Here's how the part is built. I have some questions about the finished solid (model axes, mm). Round coordinates to 2 decimals unless told otherwise and drop trailing zeros. Write each loop counter-clockwise with the first axis right and the second up, starting at its lowest first coordinate (ties: lowest second). Pieces come first, ordered by that corner, then holes. Notation, with made-up numbers: (23.25, -6) - (81.25, -6) arc R30 cw to (81.25, 27) - close; hole circle Ø8 at (84, 18.25). An arc over 180 degrees is marked (long way). One line per item, written item: value. Start each with the question number.
Item 1: Imagine slicing it at A-A, the plane y = 534. Please give me the cut outline in (x, z), then the cut area to 3 significant figures.
Item 2: For P1, Ø0.6, axis at x = 197.5, z = 0.5, coming from the +Y side; P2, Ø0.6, axis at y = 543.5, z = 1.5, coming from the -X side, each with a flat end and sliding along its axis, tell me the tip position at first contact or that it passes through.
Item 3: If I drill on line 1 (X direction, y = 539.5, z = 1.1); line 2 (X direction, y = 452.5, z = 0.6); line 3 (Y direction, x = 190.5, z = 1.75), over which ranges is the centre line in solid material (lowest first)?
```python
from build123d import *

# Parameters (mm, degrees)
EXTRUDE_1_DEPTH = 2


with BuildPart() as part:
    # 草图1 → 凸台-拉伸1 (new body)
    with BuildSketch(Plane.XY):
        with BuildLine():
            Line((244.967841267, 542.393386476), (173.531139847, 542.393386476))
            Line((173.531139847, 542.393386476), (173.531139847, 544.404513771))
            Line((173.531139847, 544.404513771), (166.427186265, 544.404513771))
            Line((166.427186265, 544.404513771), (166.427186265, 523.784577737))
            Line((166.427186265, 523.784577737), (165.125301121, 523.784577737))
            Line((165.125301121, 523.784577737), (165.381520735, 509.161664861))
            add(Edge.make_bspline(
                [(165.381520735, 509.161664861), (166.398492196, 499.581380375), (165.660716299, 482.596552628), (178.57521294, 459.918617671), (192.311763969, 447.256935323), (203.145863385, 443.111286653), (205.16102947, 442.514323356)],
                knots=[0, 0, 0, 0, 0.348658777, 0.570107959, 0.906139099, 0.980139945, 0.980139945, 0.980139945, 0.980139945], degree=3))
            Line((205.16102947, 442.514323356), (205.16102947, 472.905120341))
            Line((205.16102947, 472.905120341), (205.16102947, 474.905120341))
            Line((205.16102947, 474.905120341), (213.16329184, 474.905120341))
            Line((213.16329184, 474.905120341), (213.16329184, 472.905120341))
            Line((213.16329184, 472.905120341), (213.16329184, 442.577372397))
            add(Edge.make_bspline(
                [(253.521985396, 523.784577737), (253.388891198, 517.565791469), (253.032140526, 502.963496163), (252.103987956, 483.22463858), (243.331777802, 465.610764177), (231.612343059, 451.708919957), (219.961627576, 444.823878536), (213.16329184, 442.577372397)],
                knots=[0, 0, 0, 0, 0.186773646, 0.443708277, 0.581360863, 0.772361396, 0.983204581, 0.983204581, 0.983204581, 0.983204581], degree=3))
            Line((253.521985396, 523.784577737), (252.132324541, 523.784577737))
            Line((252.132324541, 523.784577737), (252.132324541, 544.404513771))
            Line((252.132324541, 544.404513771), (244.967841267, 544.404513771))
            Line((244.967841267, 544.404513771), (244.967841267, 542.393386476))
        make_face()
    extrude(amount=EXTRUDE_1_DEPTH)


solid = part.part
```
Values follow:
1. outline: (166.43, 0) - (252.13, 0) - (252.13, 2) - (166.43, 2) - close
1. area: 171 mm^2
2. P1: stops at y = 542.39
2. P2: stops at x = 166.43
3. line 1: x = 166.43 to 252.13
3. line 2: x = 187.49 to 205.16, 213.16 to 230.79
3. line 3: y = 450.06 to 542.39
